from build123d import *

# Parameters (mm, degrees)
F0_W          = 762
F0_H          = 9.525
F1_DEPTH      = 44.45
F2_W          = 31.75
F2_H          = 31.75
F3_DEPTH      = 25.4
F4_W          = 31.75
F4_H          = 31.75
F5_DEPTH      = 25.4
F7_DEPTH      = 762.001
F9_DEPTH      = 762.001
F10_T1_DEPTH  = 361.7347577498
F10_T3_DEPTH  = 361.7347577498
F10_T5_DEPTH  = 30.7650851852
F10_T7_DEPTH  = 30.7650851852
F10_T10_ANGLE = 27.3498757801
F10_T12_ANGLE = 27.3498757801
F10_T14_ANGLE = 27.3498757801
F10_T16_ANGLE = 27.3498757801


# Not quite as in the source:
# - a fillet or chamfer that OpenCascade refuses, or shapes differently, is made with other operations: its cross-section is extruded or revolved along the edge and cut away or added
# - a feature names something its author has since deleted; it is built from what else it names


with BuildPart() as f1:
    # F0 (on Front) → F1 (new body, symmetric)
    with BuildSketch(Plane.XZ):
        with Locations((0.726044178, 113.6916989031)):
            Rectangle(F0_W, F0_H)
        with BuildLine():
            Line((381.726044178, 108.9291989031), (-380.273955822, 108.9291989031))
            Line((-380.273955822, 108.9291989031), (-367.8846560609, 100.669665729))
            ThreePointArc((-367.8846560609, 100.669665729), (-340.9058012367, 87.0105643735), (-311.4625349518, 80.1168188064))
            Line((-311.4625349518, 80.1168188064), (0.726044178, 45.4291989031))
            Line((0.726044178, 45.4291989031), (31.5534211464, 48.8544630107))
            Line((31.5534211464, 48.8544630107), (312.9146233078, 80.1168188064))
            ThreePointArc((312.9146233078, 80.1168188064), (342.3578895927, 87.0105643735), (369.3367444169, 100.669665729))
            Line((369.3367444169, 100.669665729), (381.726044178, 108.9291989031))
        make_face()
    extrude(amount=F1_DEPTH, both=True)

    # F2 (on face) → F3 (cut)
    with BuildSketch(Plane(origin=(4.9949857842, 0, 44.954872058), x_dir=(0.9938837347, 0, -0.1104315261), z_dir=(-0.1104315261, 0, -0.9938837347))):
        with Locations((-32.870212264, 0)):
            Rectangle(F2_W, F2_H)
    extrude(amount=-F3_DEPTH, mode=Mode.SUBTRACT)

    # F4 (on face) → F5 (cut)
    with BuildSketch(Plane(origin=(-4.9772773896, 0, 44.7954965067), x_dir=(0.9938837347, 0, 0.1104315261), z_dir=(0.1104315261, 0, -0.9938837347))):
        with Locations((34.3134192624, 0)):
            Rectangle(F4_W, F4_H)
    extrude(amount=-F5_DEPTH, mode=Mode.SUBTRACT)

    # F6 (on face) → F7 (cut, through all)
    with BuildSketch(Plane.YZ.offset(381.726044178)):
        Polygon((-43.1113485495, 108.9291989031), (-44.45, 118.4541989031), (-44.45, 108.9291989031), align=None)
    extrude(amount=-F7_DEPTH, mode=Mode.SUBTRACT)

    # F8 (on face) → F9 (cut, through all)
    with BuildSketch(Plane.YZ.offset(381.726044178)):
        Polygon((44.45, 108.9291989031), (44.45, 118.4541989031), (43.1113485495, 108.9291989031), align=None)
    extrude(amount=-F9_DEPTH, mode=Mode.SUBTRACT)

    # F10: fillet of radius 6.35 on 4 edges, made by hand

    # F10_s2 → F10_t1 (cut)
    with BuildSketch(Plane(origin=(-316.457520736, 0, 35.1619467484), x_dir=(0, 1, 0), z_dir=(0.9938837347, 0, -0.1104315261))):
        with BuildLine():
            ThreePointArc((-44.45, 51.5815200356), (-42.5901280605, 47.0913919751), (-38.1, 45.2315200356))
            Line((-38.1, 45.2315200356), (-44.45, 45.2315200356))
            Line((-44.45, 45.2315200356), (-44.45, 51.5815200356))
        make_face()
        with BuildLine():
            ThreePointArc((44.45, 51.5815200356), (42.5901280605, 47.0913919751), (38.1, 45.2315200356))
            Line((38.1, 45.2315200356), (44.45, 45.2315200356))
            Line((44.45, 45.2315200356), (44.45, 51.5815200356))
        make_face()
    extrude(amount=F10_T1_DEPTH, mode=Mode.SUBTRACT)

    # F10_s4 → F10_t3 (cut)
    with BuildSketch(Plane(origin=(-41.6303912962, 0, -4.6255990329), x_dir=(0, 1, 0), z_dir=(0.9938837347, 0, 0.1104315261))):
        with BuildLine():
            ThreePointArc((-44.45, 51.4211637025), (-42.5901280605, 46.9310356419), (-38.1, 45.0711637025))
            Line((-38.1, 45.0711637025), (-44.45, 45.0711637025))
            Line((-44.45, 45.0711637025), (-44.45, 51.4211637025))
        make_face()
        with BuildLine():
            ThreePointArc((44.45, 51.4211637025), (42.5901280605, 46.9310356419), (38.1, 45.0711637025))
            Line((38.1, 45.0711637025), (44.45, 45.0711637025))
            Line((44.45, 45.0711637025), (44.45, 51.4211637025))
        make_face()
    extrude(amount=F10_T3_DEPTH, mode=Mode.SUBTRACT)

    # F10_s6 → F10_t5 (cut)
    with BuildSketch(Plane(origin=(-326.7503981008, 0, 217.8335987339), x_dir=(0, 1, 0), z_dir=(0.8320502943, 0, -0.5547001962))):
        with BuildLine():
            ThreePointArc((38.1, -120.3034659045), (42.5901280605, -118.443593965), (44.45, -113.9534659045))
            Line((44.45, -113.9534659045), (44.45, -120.3034659045))
            Line((44.45, -120.3034659045), (38.1, -120.3034659045))
        make_face()
        with BuildLine():
            ThreePointArc((-38.1, -120.3034659045), (-42.5901280605, -118.443593965), (-44.45, -113.9534659045))
            Line((-44.45, -113.9534659045), (-44.45, -120.3034659045))
            Line((-44.45, -120.3034659045), (-38.1, -120.3034659045))
        make_face()
    extrude(amount=F10_T5_DEPTH, mode=Mode.SUBTRACT)

    # F10_s8 → F10_t7 (cut)
    with BuildSketch(Plane(origin=(302.1575918559, 0, 201.4383945706), x_dir=(0, 1, 0), z_dir=(0.8320502943, 0, 0.5547001962))):
        with BuildLine():
            ThreePointArc((44.45, -114.7589396005), (42.5901280605, -119.2490676611), (38.1, -121.1089396005))
            Line((38.1, -121.1089396005), (44.45, -121.1089396005))
            Line((44.45, -121.1089396005), (44.45, -114.7589396005))
        make_face()
        with BuildLine():
            ThreePointArc((-44.45, -114.7589396005), (-42.5901280605, -119.2490676611), (-38.1, -121.1089396005))
            Line((-38.1, -121.1089396005), (-44.45, -121.1089396005))
            Line((-44.45, -121.1089396005), (-44.45, -114.7589396005))
        make_face()
    extrude(amount=F10_T7_DEPTH, mode=Mode.SUBTRACT)

    # F10_s9 → F10_t10 (revolve, cut)
    with BuildSketch(Plane(origin=(-301.1522999171, 0, 200.7681999448), x_dir=(0, 1, 0), z_dir=(-0.8320502943, 0, 0.5547001962))):
        with BuildLine():
            ThreePointArc((44.45, 113.9534659045), (42.5901280605, 118.443593965), (38.1, 120.3034659045))
            Line((38.1, 120.3034659045), (44.45, 120.3034659045))
            Line((44.45, 120.3034659045), (44.45, 113.9534659045))
        make_face()
    revolve(axis=Axis((-297.4377311403, 44.45, 206.34005311), (0, -1, 0)), revolution_arc=F10_T10_ANGLE, mode=Mode.SUBTRACT)

    # F10_s11 → F10_t12 (revolve, cut)
    with BuildSketch(Plane(origin=(317.8919006975, 0, 35.3213222997), x_dir=(0, 1, 0), z_dir=(-0.9938837347, 0, -0.1104315261))):
        with BuildLine():
            ThreePointArc((44.45, -51.4211637025), (42.5901280605, -46.9310356419), (38.1, -45.0711637025))
            Line((38.1, -45.0711637025), (44.45, -45.0711637025))
            Line((44.45, -45.0711637025), (44.45, -51.4211637025))
        make_face()
    revolve(axis=Axis((298.8898194963, 44.45, 206.34005311), (0, -1, 0)), revolution_arc=F10_T12_ANGLE, mode=Mode.SUBTRACT)

    # F10_s13 → F10_t14 (revolve, cut)
    with BuildSketch(Plane(origin=(317.8919006975, 0, 35.3213222997), x_dir=(0, 1, 0), z_dir=(-0.9938837347, 0, -0.1104315261))):
        with BuildLine():
            ThreePointArc((-44.45, -51.4211637025), (-42.5901280605, -46.9310356419), (-38.1, -45.0711637025))
            Line((-38.1, -45.0711637025), (-44.45, -45.0711637025))
            Line((-44.45, -45.0711637025), (-44.45, -51.4211637025))
        make_face()
    revolve(axis=Axis((298.8898194963, -44.45, 206.34005311), (0, -1, 0)), revolution_arc=F10_T14_ANGLE, mode=Mode.SUBTRACT)

    # F10_s15 → F10_t16 (revolve, cut)
    with BuildSketch(Plane(origin=(-301.1522999171, 0, 200.7681999448), x_dir=(0, 1, 0), z_dir=(-0.8320502943, 0, 0.5547001962))):
        with BuildLine():
            ThreePointArc((-38.1, 120.3034659045), (-42.5901280605, 118.443593965), (-44.45, 113.9534659045))
            Line((-44.45, 113.9534659045), (-44.45, 120.3034659045))
            Line((-44.45, 120.3034659045), (-38.1, 120.3034659045))
        make_face()
    revolve(axis=Axis((-297.4377311403, -44.45, 206.34005311), (0, -1, 0)), revolution_arc=F10_T16_ANGLE, mode=Mode.SUBTRACT)


solid = f1.part
Could you check a few things on this model? Use its own coordinates, in mm. A direction names the side the tool comes from. Coordinates: 2 decimals unless noted, no trailing zeros. Write each loop counter-clockwise with the first axis right and the second up, starting at its lowest first coordinate (ties: lowest second). Pieces come first, ordered by that corner, then holes. Notation, with made-up numbers: M 37,88 L 68,88 A26 cw 68,113 Z; hole C 36,20 d6. An arc over 180 degrees is marked long. One line per question, with ' | ' between items.
1) For faces 1 (the face through (-42.07, 0.22, 62.78)), 2 (the face through (154.64, -0.53, 62.53)), which set-ups out of +Z, -Z, +X, -X, +Y, -Y let a thin tool reach every point of the face, with its end or its side?
Checks:
face 1: -Z | face 2: -Z, +X, +Y, -Y
2) For pin 1 Ø23 at (x, z) = (35.5, 54.5) entering from -Y; pin 2 Ø1.5 at (x, y) = (-114, -15) entering from -Z; pin 3 Ø5 at (y, z) = (-15, 104.5) entering from +X; pin 4 Ø1.5 at (y, z) = (-18, 102) entering from -X, each with a flat end and sliding along its axis, tell me the tip position at first contact or that it passes through.
Checks:
pin 1: y = -44.45 | pin 2: z = 58.09 | pin 3: x = 378.83 | pin 4: x = -371.01
3) Imagine slicing it at B-B, the plane y = -29. Write out the boundary of the cut face in (x, z), and give its area (3 significant figures).
Checks:
outline: M -380.27,108.93 L -367.88,100.67 A127 ccw -311.46,80.12 L 0.73,45.43 L 312.91,80.12 A127 ccw 369.34,100.67 L 381.73,108.93 L 381.73,118.45 L -380.27,118.45 Z | area: 38,600 mm²
4) Imagine slicing it at A-A, the plane y = 1.5. Write out the boundary of the cut face in (x, z), and give its area (3 significant figures).
Checks:
outline: M -380.27,108.93 L -367.88,100.67 A127 ccw -311.46,80.12 L -43.45,50.34 L -40.65,75.58 L -9.09,72.08 L -11.9,46.83 L 0.73,45.43 L 13.35,46.83 L 10.54,72.08 L 42.1,75.58 L 44.9,50.34 L 312.91,80.12 A127 ccw 369.34,100.67 L 381.73,108.93 L 381.73,118.45 L -380.27,118.45 Z | area: 36,900 mm²
5) If we mould it in two halves opening along X, with no side actions, what happens to faces 3 (the face through (154.42, -42.64, 64.43)), 4 (the face through (-4, -44.45, 87)), 5 (the face through (-27, -15.875, 61)), 6 (the face through (43.52, 0.22, 62.78))? For each: released by +X, released by -X, zero draft, split by the parting line, or undercut.
Checks:
face 3: released by +X | face 4: zero draft | face 5: undercut | face 6: undercut
6) I need wall thicknesses on probe 1 along Y at (x, z) = (8.5, 109); probe 2 along Y at (x, z) = (-65, 113); probe 3 along Z at (x, y) = (224.5, -16.5). Which ranges of each line are inside material? Lowest first, please. Write a range as [from, to].
Checks:
probe 1: [-43.12, 43.12] | probe 2: [-43.68, 43.68] | probe 3: [70.29, 118.45]
